Here's how the part is built. I have some questions about the finished solid (model axes, mm). Face numbers are marked on the shaded views. A direction names the side the tool comes from. Round coordinates to 2 decimals unless told otherwise and drop trailing zeros. Write each loop counter-clockwise with the first axis right and the second up, starting at its lowest first coordinate (ties: lowest second). Pieces come first, ordered by that corner, then holes. Notation, with made-up numbers: (84, 76) - (118, 76) arc R12 ccw to (118, 87) - close; hole circle Ø1 at (50, -11.75). An arc over 180 degrees is marked (long way). Write item = value, one per line. Start each with the question number.
Item 1: Which directions (+Z, -Z, +X, -X, +Y, -Y) give clear straight access to the entire face, cutting with the end or side of a thin tool? Please do the marked faces 1 and 2.
Item 2: If I drill on line 1 along Y through (x, z) = (-28, 5.25); line 2 along Y through (x, z) = (1, 7.25); line 3 along Z through (x, y) = (-4, 28.5), over which ranges is the centre line in solid material (lowest first)? Write a range as [from, to].
Item 3: If we section it at C-C (y = 20): Please give me the cut outline in (x, z), and give its area (3 significant figures).
Item 4: Thinking about a two-plate mould opening in Y: for the marked faces 3, 4, 5 and 6, which applies, pulls with the +Y half, pulls with the -Y half, needs draft (parallel to the pull), parting line crosses it, or undercut?
Item 5: For P1, Ø7, axis at x = -26.18, y = -28.86, coming from the +Z side; P2, Ø8.5, axis at x = -1.18, y = -21.86, coming from the -Z side, each with a flat end and sliding along its axis, tell me the tip position at first contact or that it passes through.
Item 6: If we section it at A-A (y = -21): Please give me the cut outline in (x, z).
Item 7: If we section it at D-D (x = -5.5): Please give me the cut outline in (y, z), and give its area (3 significant figures).
Item 8: If we section it at B-B (z = 6): Please give me the cut outline in (x, y), and give its area (3 significant figures).
```python
from build123d import *

# Parameters (mm, degrees)
ESQUISSE1_W             = 45
ESQUISSE1_H             = 80
ESQUISSE1_R             = 3.3
ESQUISSE1_R_2           = 2.75
BOSS_EXTRU_1_DEPTH      = 10
ESQUISSE2_R             = 6
ENL_V_MAT_EXTRU_1_DEPTH = 5
ESQUISSE3_R             = 7
ENL_V_MAT_EXTRU_3_DEPTH = 7


with BuildPart() as part:
    # Esquisse1 → Boss.-Extru.1 (new body)
    with BuildSketch(Plane.XY):
        with Locations((-13.678136106, 1.138047212)):
            Rectangle(ESQUISSE1_W, ESQUISSE1_H)
        with Locations((-1.178136106, 24.138047212)):
            Circle(ESQUISSE1_R, mode=Mode.SUBTRACT)
        with Locations((-1.178136106, -21.861952788)):
            Circle(ESQUISSE1_R, mode=Mode.SUBTRACT)
        with Locations((-26.178136106, 31.138047212)):
            Circle(ESQUISSE1_R_2, mode=Mode.SUBTRACT)
        with Locations((-26.178136106, -28.861952788)):
            Circle(ESQUISSE1_R_2, mode=Mode.SUBTRACT)
    extrude(amount=BOSS_EXTRU_1_DEPTH)

    # Esquisse2 → Enlèv. mat.-Extru.1 (cut)
    with BuildSketch(Plane.XY.offset(10)):
        with Locations((-26.178136106, 31.138047212)):
            Circle(ESQUISSE2_R)
        with Locations((-26.178136106, -28.861952788)):
            Circle(ESQUISSE2_R)
    extrude(amount=-ENL_V_MAT_EXTRU_1_DEPTH, mode=Mode.SUBTRACT)

    # Esquisse3 → Enlèv. mat.-Extru.3 (cut)
    with BuildSketch(Plane(origin=(0, 0, 0), x_dir=(-1, 0, 0), z_dir=(0, 0, -1))):
        with Locations((1.178136106, 24.138047212)):
            Circle(ESQUISSE3_R)
        with Locations((1.178136106, -21.861952788)):
            Circle(ESQUISSE3_R)
    extrude(amount=-ENL_V_MAT_EXTRU_3_DEPTH, mode=Mode.SUBTRACT)


solid = part.part
```
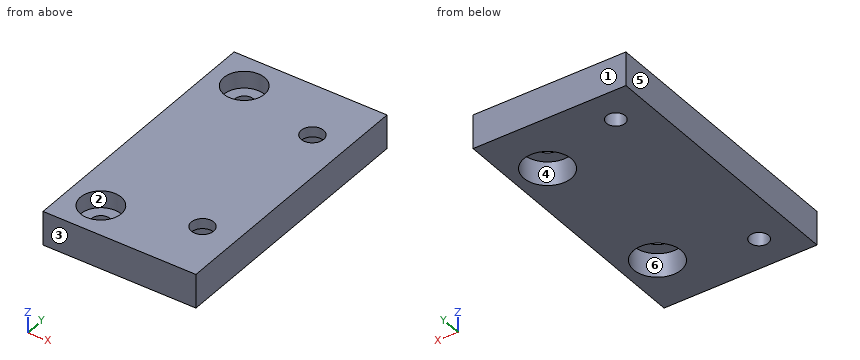
Reply:
q1.face_1 = +Z, -Z, +X, -X, +Y
q1.face_2 = +Z
q2.line_1 = [-38.86, -34.58], [-23.15, 25.42], [36.85, 41.14]
q2.line_2 = [-38.86, -24.34], [-19.38, 21.66], [26.62, 41.14]
q2.line_3 = [7, 10]
q3.outline = (-36.18, 0) - (-6.82, 0) - (-6.82, 7) - (4.47, 7) - (4.47, 0) - (8.82, 0) - (8.82, 10) - (-36.18, 10) - close
q3.area = 371 mm2
q4.face_3 = pulls with the -Y half
q4.face_4 = undercut
q4.face_5 = needs draft
q4.face_6 = undercut
q5.P1 = 5
q5.P2 = 7
q6.outline = (-36.18, 0) - (-8.12, 0) - (-8.12, 7) - (-4.36, 7) - (-4.36, 10) - (-36.18, 10) - close; (2.01, 7) - (5.77, 7) - (5.77, 0) - (8.82, 0) - (8.82, 10) - (2.01, 10) - close
q7.outline = (-38.86, 0) - (-27.37, 0) - (-27.37, 7) - (-16.36, 7) - (-16.36, 0) - (18.63, 0) - (18.63, 7) - (29.64, 7) - (29.64, 0) - (41.14, 0) - (41.14, 10) - (-38.86, 10) - close
q7.area = 646 mm2
q8.outline = (-36.18, -38.86) - (8.82, -38.86) - (8.82, 41.14) - (-36.18, 41.14) - close; hole circle Ø12 at (-26.18, -28.86); hole circle Ø12 at (-26.18, 31.14); hole circle Ø14 at (-1.18, -21.86); hole circle Ø14 at (-1.18, 24.14)
q8.area = 3,070 mm2
